```python
from build123d import *

# Parameters (mm, degrees)
SKETCH1_W           = 50
SKETCH1_H           = 30
BOSS_EXTRUDE1_DEPTH = 1.5
SKETCH2_R           = 1.75
CUT_EXTRUDE1_DEPTH  = 2.5
SKETCH3_W           = 2
SKETCH3_H           = 13
BOSS_EXTRUDE2_DEPTH = 8
SKETCH4_W           = 12
SKETCH4_H           = 6
BOSS_EXTRUDE3_DEPTH = 5
SKETCH5_R           = 2.5
BOSS_EXTRUDE4_DEPTH = 2
SKETCH6_W           = 6
SKETCH6_H           = 7
BOSS_EXTRUDE5_DEPTH = 1.8


with BuildPart() as part:
    # Sketch1 → Boss-Extrude1 (new body)
    with BuildSketch(Plane(origin=(0, 0, 0), x_dir=(1, 0, 0), z_dir=(0, 1, 0))):
        with Locations((25, -15)):
            Rectangle(SKETCH1_W, SKETCH1_H)
    extrude(amount=BOSS_EXTRUDE1_DEPTH)

    # Sketch2 → Cut-Extrude1 (cut, through all)
    with BuildSketch(Plane(origin=(0, 1.5, 0), x_dir=(1, 0, 0), z_dir=(0, 1, 0))):
        with Locations((48, -28)):
            Circle(SKETCH2_R)
        with Locations((48, -2)):
            Circle(SKETCH2_R)
        with Locations((2, -2)):
            Circle(SKETCH2_R)
        with Locations((2, -28)):
            Circle(SKETCH2_R)
    extrude(amount=-CUT_EXTRUDE1_DEPTH, mode=Mode.SUBTRACT)

    # Sketch3 → Boss-Extrude2 (add)
    with BuildSketch(Plane(origin=(0, 1.5, 0), x_dir=(1, 0, 0), z_dir=(0, 1, 0))):
        with Locations((48, -15)):
            Rectangle(SKETCH3_W, SKETCH3_H)
    extrude(amount=BOSS_EXTRUDE2_DEPTH)

    # Sketch4 → Boss-Extrude3 (add)
    with BuildSketch(Plane(origin=(0, 1.5, 0), x_dir=(1, 0, 0), z_dir=(0, 1, 0))):
        with Locations((6, -21.5)):
            Rectangle(SKETCH4_W, SKETCH4_H)
    extrude(amount=BOSS_EXTRUDE3_DEPTH)

    # Sketch5 → Boss-Extrude4 (add)
    with BuildSketch(Plane.ZY):
        with Locations((21.5, 4)):
            Circle(SKETCH5_R)
    extrude(amount=BOSS_EXTRUDE4_DEPTH)

    # Sketch6 → Boss-Extrude5 (add)
    with BuildSketch(Plane(origin=(0, 1.5, 0), x_dir=(1, 0, 0), z_dir=(0, 1, 0))):
        with Locations((1, -9.7)):
            Rectangle(SKETCH6_W, SKETCH6_H)
    extrude(amount=BOSS_EXTRUDE5_DEPTH)


solid = part.part
```
Build history of the part. All positions in model axes, mm. A direction names the side the tool comes from. Coordinates: 2 decimals unless noted, no trailing zeros. Write each loop counter-clockwise with the first axis right and the second up, starting at its lowest first coordinate (ties: lowest second). Pieces come first, ordered by that corner, then holes.
1. Pull direction X, two halves, no side cores. Call faces 6 (the flat face through (6, 6.5, 21)), 7 (the flat face through (50, 1, 15)), 8 (the flat face through (-2, 2, 10)), 9 (the cylindrical face through (49.669, 0.76, 27.474)): released by +X, released by -X, zero draft, split by the parting line, or undercut.
Answer block:
face 6: zero draft
face 7: released by +X
face 8: released by -X
face 9: undercut
2. 3-axis set-ups, long thin cutter, end or side, ignore diameter. For faces 1 (the flat face through (48, 5, 8.5)), 2 (the flat face through (47, 5, 15)), 3 (the flat face through (6, 4, 24.5)), 4 (the cylindrical face through (-1, 4, 19)), 5 (the flat face through (-1, 1.5, 10)): which of +Z, -Z, +X, -X, +Y, -Y reach the whole face in a straight line?
Answer block:
face 1: -Z, +X, +Y
face 2: +Z, -Z, +Y
face 3: +Z, +X, -X, +Y
face 4: -X
face 5: +Z, -Z, -X, -Y
3. Band-saw the part on C-C, the plane z = 28. Give the cut face in (x, y).
Answer block:
outline: (0, 0) - (0.25, 0) - (0.25, 1.5) - (0, 1.5) - close; (3.75, 0) - (46.25, 0) - (46.25, 1.5) - (3.75, 1.5) - close; (49.75, 0) - (50, 0) - (50, 1.5) - (49.75, 1.5) - close
4. Band-saw the part on D-D, the plane x = 48. Give the cut face in (y, z), and give its area (4 significant figures).
Answer block:
outline: (0, 0) - (1.5, 0) - (1.5, 0.25) - (0, 0.25) - close; (0, 3.75) - (1.5, 3.75) - (1.5, 8.5) - (9.5, 8.5) - (9.5, 21.5) - (1.5, 21.5) - (1.5, 26.25) - (0, 26.25) - close; (0, 29.75) - (1.5, 29.75) - (1.5, 30) - (0, 30) - close
area: 138.5 mm2
5. Drill centre lines: probe 1 along Z at (x, y) = (2, 0.3); probe 2 along X at (y, z) = (1.2, 28); probe 3 along X at (y, z) = (3.25, 11). Where is each one in solid material? Low to high.
Answer block:
probe 1: z = 0 to 0.25, 3.75 to 26.25, 29.75 to 30
probe 2: x = 0 to 0.25, 3.75 to 46.25, 49.75 to 50
probe 3: x = -2 to 4, 47 to 49
6. Band-saw the part on A-A, the plane y = 6. Give the cut face in (x, z).
Answer block:
outline: (-2, 20) - (0, 20) - (0, 18.5) - (12, 18.5) - (12, 24.5) - (0, 24.5) - (0, 23) - (-2, 23) - close; (47, 8.5) - (49, 8.5) - (49, 21.5) - (47, 21.5) - close
7. Drop flat-ended pins along their axis: pin 1 (2 mm diameter, centred on x = 48, z = 28, fed in from -Y); pin 2 (1.4 mm diameter, centred on y = 2.5, z = 10, fed in from +X); pin 3 (0.6 mm diameter, centred on x = 47.5, y = 4.5, fed in from -Z); pin 4 (4 mm diameter, centred on x = 32.5, z = 6.5, fed in from +Y). Give the stop position or say it passes through.
Answer block:
pin 1: passes through
pin 2: stops at x = 49
pin 3: stops at z = 8.5
pin 4: stops at y = 1.5
8. Band-saw the part on B-B, the plane x = 2. Give the cut face in (y, z).
Answer block:
outline: (0, 0) - (1.5, 0) - (1.5, 0.25) - (0, 0.25) - close; (0, 3.75) - (1.5, 3.75) - (1.5, 6.2) - (3.3, 6.2) - (3.3, 13.2) - (1.5, 13.2) - (1.5, 18.5) - (6.5, 18.5) - (6.5, 24.5) - (1.5, 24.5) - (1.5, 26.25) - (0, 26.25) - close; (0, 29.75) - (1.5, 29.75) - (1.5, 30) - (0, 30) - close
